```python
from build123d import *

# Parameters (mm, degrees)
SKETCH1_R           = 1.8288
SKETCH1_R_2         = 4.7625
BOSS_EXTRUDE1_DEPTH = 3.175
CUT_EXTRUDE1_DEPTH  = 57.415004653
FILLET1_R           = 2.5
FILLET2_R           = 5


with BuildPart() as part:
    # Sketch1 → Boss-Extrude1 (new body)
    with BuildSketch(Plane(origin=(0, 0, 0), x_dir=(0, 0, -1), z_dir=(1, 0, 0))):
        with BuildLine():
            Line((-16.645, -53.81), (16.645, -53.81))
            Line((16.645, -53.81), (16.645, 5.15))
            Line((16.645, 5.15), (6.94973031, 37.108353593))
            ThreePointArc((6.94973031, 37.108353593), (0, 42.2625), (-6.94973031, 37.108353593))
            Line((-6.94973031, 37.108353593), (-16.645, 5.15))
            Line((-16.645, 5.15), (-16.645, -53.81))
        make_face()
        with Locations((-13.4747, 0)):
            Circle(SKETCH1_R, mode=Mode.SUBTRACT)
        with Locations((0, 35)):
            Circle(SKETCH1_R_2, mode=Mode.SUBTRACT)
        with Locations((13.4747, 0)):
            Circle(SKETCH1_R, mode=Mode.SUBTRACT)
        with Locations((-13.4747, -50)):
            Circle(SKETCH1_R, mode=Mode.SUBTRACT)
        with Locations((13.4747, -50)):
            Circle(SKETCH1_R, mode=Mode.SUBTRACT)
    extrude(amount=BOSS_EXTRUDE1_DEPTH)

    # Sketch2 → Cut-Extrude1 (cut, through all)
    with BuildSketch(Plane(origin=(3.175, 0, 0), x_dir=(0, 0, -1), z_dir=(1, 0, 0))):
        Polygon((11.645, -5.219501679), (1.407493202, -25), (11.645, -44.780498321), align=None)
        Polygon((0, -27.719501679), (-10.237506798, -47.5), (10.237506798, -47.5), align=None)
        Polygon((-11.645, -5.219501679), (-11.645, -44.780498321), (-1.407493202, -25), align=None)
        Polygon((-10.237506798, -2.5), (0, -22.280498321), (10.237506798, -2.5), align=None)
    extrude(amount=-CUT_EXTRUDE1_DEPTH, mode=Mode.SUBTRACT)

    # Fillet1
    fillet1_edges = [part.edges().sort_by_distance(p)[0] for p in [
        (1.5875, -44.780498321, 11.645),
        (1.5875, -5.219501679, 11.645),
        (1.5875, -25, 1.407493202),
        (1.5875, -47.5, -10.237506798),
        (1.5875, -47.5, 10.237506798),
        (1.5875, -27.719501679, 0),
        (1.5875, -22.280498321, 0),
        (1.5875, -2.5, 10.237506798),
        (1.5875, -2.5, -10.237506798),
        (1.5875, -25, -1.407493202),
        (1.5875, -5.219501679, -11.645),
        (1.5875, -44.780498321, -11.645),
    ]]
    fillet(fillet1_edges, radius=FILLET1_R)

    # Fillet2
    fillet2_edges = [part.edges().sort_by_distance(p)[0] for p in [
        (1.5875, -53.81, -16.645),
        (1.5875, -53.81, 16.645),
        (1.5875, 5.15, 16.645),
        (1.5875, 5.15, -16.645),
    ]]
    fillet(fillet2_edges, radius=FILLET2_R)


solid = part.part
```
Work out the finished part from the listing and answer in its coordinate system (mm). A direction names the side the tool comes from. Give positions to 0.01 mm unless a question says otherwise; leave off trailing zeros. Order: outer loops, then holes, each group sorted by start corner. A loop starts at its lowest first (then second) coordinate and runs counter-clockwise, first axis right, second up. Notation, with made-up numbers: (86.5, -27) -> (107.5, -27) arc R13 cw to (107.5, -21) -> close; hole circle Ø5 at (-30, 13.25). An arc over 180 degrees is marked (long way). Answer as CSV lines item,"result". Start each with the question number.
(1) Section B-B, the plane y = 0 is taken. Write down the section's boundary in (x, z) (1 decimal).
(2) Which of the six approach directions +Z, -Z, +X, -X, +Y, -Y give full straight-line access (tool end or side, diameter ignored) to faces 1 (the cylindrical face through (1.57, 42.26, -0.13)), 2 (the flat face through (1.61, -38.013, -5.327))?
(3) Section D-D, the plane y = 35 is taken. Write down the section's boundary in (x, z) (1 decimal), plus the area to 3 significant figures.
(4) This flat-tipped pin is pushed along its axis until it touches: pin 1 Ø3 at (y, z) = (-50, 13.47) entering from -X. Where does it stop, or does it pass through?
(5) Section A-A, the plane z = 0 is taken. Write down the section's boundary in (x, y) (1 decimal), plus the area to 3 significant figures.
(6) Section C-C, the plane z = -13.5 is taken. Write down the section's boundary in (x, y) (3 decimals).
(7) For a pull along Z with two mould halves and no side action, classify faces 3 (the cylindrical face through (1.57, -36.93, 9.78)), 4 (the cylindrical face through (1.61, -52.384, -15.141)), 5 (the flat face through (0, -16, 4)) as released by +Z, released by -Z, zero draft, split by the parting line, or undercut.
(8) Consider line 1 along Y through (x, z) = (2.35, 0); line 2 along Y through (x, z) = (2.05, 1); line 3 along Y through (x, z) = (3, 2). Determine where each line is inside the solid, lowest interval first.
Entries:
1,outline,"(0, -16.6) -> (3.2, -16.6) -> (3.2, -15.3) -> (0, -15.3) -> close; (0, -11.6) -> (3.2, -11.6) -> (3.2, 11.6) -> (0, 11.6) -> close; (0, 15.3) -> (3.2, 15.3) -> (3.2, 16.6) -> (0, 16.6) -> close"
2,face 1,"+X, -X, +Y"
2,face 2,"+X, -X"
3,outline,"(0, -7.6) -> (3.2, -7.6) -> (3.2, -4.8) -> (0, -4.8) -> close; (0, 4.8) -> (3.2, 4.8) -> (3.2, 7.6) -> (0, 7.6) -> close"
3,area,"18.0 mm²"
4,pin 1,"through"
5,outline,"(0, -53.8) -> (3.2, -53.8) -> (3.2, -47.5) -> (0, -47.5) -> close; (0, -30.7) -> (3.2, -30.7) -> (3.2, -19.3) -> (0, -19.3) -> close; (0, -2.5) -> (3.2, -2.5) -> (3.2, 30.2) -> (0, 30.2) -> close; (0, 39.8) -> (3.2, 39.8) -> (3.2, 42.3) -> (0, 42.3) -> close"
5,area,"168 mm²"
6,outline,"(0, -53.453) -> (3.175, -53.453) -> (3.175, -51.829) -> (0, -51.829) -> close; (0, -48.171) -> (3.175, -48.171) -> (3.175, -1.829) -> (0, -1.829) -> close; (0, 1.829) -> (3.175, 1.829) -> (3.175, 15.517) -> (0, 15.517) -> close"
7,face 3,"undercut"
7,face 4,"released by -Z"
7,face 5,"zero draft"
8,line 1,"-53.81 to -47.5, -30.66 to -19.34, -2.5 to 30.24, 39.76 to 42.26"
8,line 2,"-53.81 to -47.5, -30.87 to -19.13, -2.5 to 30.34, 39.66 to 42.19"
8,line 3,"-53.81 to -47.5, -31.66 to -26.14, -23.86 to -18.34, -2.5 to 30.68, 39.32 to 41.98"
